Autodesk Fusion 360 part; units mm, degrees
sketch "Sketch1" plane through (0, 0, 0) normal (0, 1, 0) x (1, 0, 0)
  line L0 (-31.5, 5) -> (33.3053, 5)
  line L1 (33.3053, 5) -> (33.3053, -5)
  line L2 (33.3053, -5) -> (-31.5, -5)
  line L3 (-31.5, -5) -> (-31.5, 5)
  line L4 (-31.5, 0) -> (-36.5072, 0) construction
  line L5 (1.75, 0) -> (22.5, 0) construction
  point P0 (-26, 0)
  point P1 (-19, 0)
  point P2 (-12, 0)
  point P3 (-5, 0)
  point P4 (-31.5, 0)
  dimension "d6" = 7
  dimension "d7" = 0
  dimension "d21" = 5
  dimension "d22" = 5.5
  dimension "d23" = 10
extrude "Extrude1" add sketch "Sketch1" along normal blind 7.5
hole "Hole1" at (-26, 0, 0) direction (0, 1, 0) diameter 3 end up to surface (7.5 mm away)
hole "Hole2" at (-19, 0, 0) direction (0, 1, 0) diameter 3.1 end up to surface (7.5 mm away)
hole "Hole3" at (-12, 0, 0) direction (0, 1, 0) diameter 3.2 end up to surface (7.5 mm away)
hole "Hole4" at (-5, 0, 0) direction (0, 1, 0) diameter 3.3 end up to surface (7.5 mm away)
mirror "Mirror1" about plane through (0, 0, 0) normal (1, 0, 0) of "Hole4", "Hole3", "Hole2", "Hole1"
Input: part model. Units: mm. Frame: model coordinates. Give positions to 0.01 mm unless a question says otherwise; leave off trailing zeros. Order: outer loops, then holes, each group sorted by start corner. A loop starts at its lowest first (then second) coordinate and runs counter-clockwise, first axis right, second up. Notation, with made-up numbers: (-18.5, 89.5) - (17.5, 89.5) arc R19 ccw to (17.5, 104.5) - close; hole circle Ø5 at (72.5, -33). An arc over 180 degrees is marked (long way). One line per item, written item: value.
1. Draft query along X for faces 1 (the face through (33.305, 4, 0)), 2 (the face through (13.56, 3.8, 0.35)), 3 (the face through (0, 4, -5)), 4 (the face through (-13.586, 3.802, 0.208)). Return one class per face: released by +X, released by -X, zero draft, split by the parting line, or undercut.
Determined:
face 1: released by +X
face 2: undercut
face 3: zero draft
face 4: undercut
2. Cut plane A-A, the plane x = -19. Output: boundary loops of the cut face in (y, z).
Determined:
outline: (0, -5) - (7.5, -5) - (7.5, -1.55) - (0, -1.55) - close; (0, 1.55) - (7.5, 1.55) - (7.5, 5) - (0, 5) - close
3. Cut plane B-B, the plane y = 4.25. Give the number of separate pieces and of enclosed holes in the cut face, and give its area (3 significant figures).
Determined:
separate pieces: 1
enclosed holes: 8
area: 586 mm2
4. Pin query (flat end, axial travel): pin 1 Ø4.5 at (x, z) = (-5, 0) entering from -Y. Return the tip coordinate at first contact, or that it passes through.
Determined:
pin 1: y = 0
5. Line query: probe 1 along Z at (x, y) = (-19, 3.75). Output: solid intervals per line, ascending.
Determined:
probe 1: -5 to -1.55, 1.55 to 5
6. Cut plane C-C, the plane x = 12. Output: boundary loops of the cut face in (y, z).
Determined:
outline: (0, -5) - (7.5, -5) - (7.5, -1.6) - (0, -1.6) - close; (0, 1.6) - (7.5, 1.6) - (7.5, 5) - (0, 5) - close
